Check sheet for the drawn part. Datum: minimum x, y, z corner. Units: mm. Round coordinates to 2 decimals unless told otherwise and drop trailing zeros. Write each loop counter-clockwise with the first axis right and the second up, starting at its lowest first coordinate (ties: lowest second). Pieces come first, ordered by that corner, then holes. Notation, with made-up numbers: (18, -7) - (65, -7) arc R19 cw to (65, 16) - close; hole circle Ø1 at (78, 26.5). An arc over 180 degrees is marked (long way). Write each question's results on one line, items separated by ' | '.
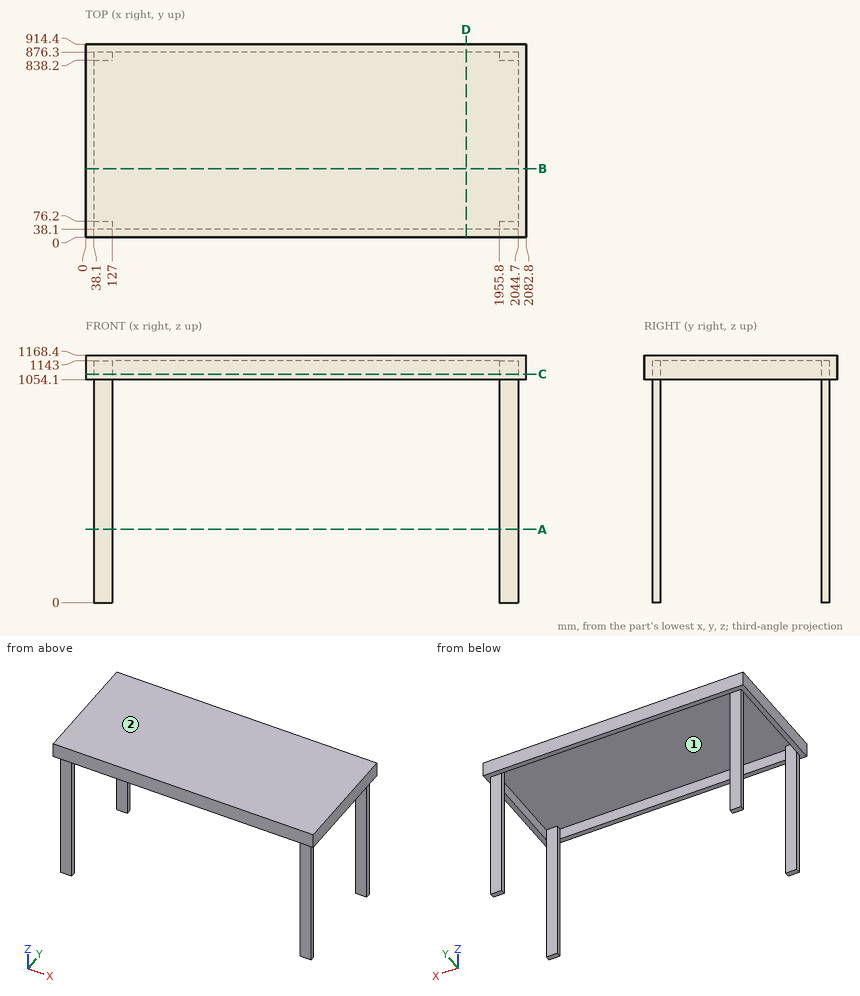
(1) Section check A-A (z = 345.5). Record the cut outline in (x, y), plus the area to 3 significant figures.
Answer:
outline: (38.1, 38.1) - (127, 38.1) - (127, 76.2) - (38.1, 76.2) - close; (38.1, 838.2) - (127, 838.2) - (127, 876.3) - (38.1, 876.3) - close; (1955.8, 38.1) - (2044.7, 38.1) - (2044.7, 76.2) - (1955.8, 76.2) - close; (1955.8, 838.2) - (2044.7, 838.2) - (2044.7, 876.3) - (1955.8, 876.3) - close | area: 13,500 mm2
(2) Section check B-B (y = 325.5). Record the cut outline in (x, z).
Answer:
outline: (0, 1054.1) - (38.1, 1054.1) - (38.1, 1143) - (2044.7, 1143) - (2044.7, 1054.1) - (2082.8, 1054.1) - (2082.8, 1168.4) - (0, 1168.4) - close
(3) Thickness scan on L1, parallel to Y at x = 1997.5, z = 320.5; L2, parallel to X at y = 299.5, z = 1112.5; L3, parallel to Z at x = 973, y = 210.5. Record the ranges inside material, lowest first.
Answer:
L1: 38.1 to 76.2, 838.2 to 876.3 | L2: 0 to 38.1, 2044.7 to 2082.8 | L3: 1143 to 1168.4
(4) Mould release check, pull along Y, two halves, no side actions. Record for the marked faces 1 and 2: released by +Y, released by -Y, zero draft, split by the parting line, or undercut.
Answer:
face 1: undercut | face 2: zero draft
(5) Section check D-D (x = 1799). Record the cut outline in (y, z).
Answer:
outline: (0, 1054.1) - (38.1, 1054.1) - (38.1, 1143) - (876.3, 1143) - (876.3, 1054.1) - (914.4, 1054.1) - (914.4, 1168.4) - (0, 1168.4) - close
(6) Go/stop test with a flat-tipped pin: pin 1 Ø19 at (y, z) = (862.5, 636.5) entering from +X. Record where the tip stops, or that it passes through.
Answer:
pin 1: x = 2044.7
(7) Section check C-C (z = 1080.5). Record the cut outline in (x, y), plus the area to 3 significant figures.
Answer:
outline: (0, 0) - (2082.8, 0) - (2082.8, 914.4) - (0, 914.4) - close; hole (38.1, 76.2) - (127, 76.2) - (127, 38.1) - (1955.8, 38.1) - (1955.8, 76.2) - (2044.7, 76.2) - (2044.7, 838.2) - (1955.8, 838.2) - (1955.8, 876.3) - (127, 876.3) - (127, 838.2) - (38.1, 838.2) - close | area: 236,000 mm2
